from build123d import *

# Parameters (mm, degrees)
SKETCH_1_R             = 7
EXTRUDE_1_DEPTH        = 160
EXTRUDE_1_DEPTH_BACK   = 36
SKETCH_2_R             = 7
EXTRUDE_2_DEPTH        = 8
SKETCH_3_W             = 18
SKETCH_3_H             = 11
EXTRUDE_3_DEPTH        = 15
EXTRUDE_4_DEPTH        = 30
SKETCH_5_W             = 60
SKETCH_5_H             = 40
EXTRUDE_5_DEPTH        = 6
SKETCH_6_W             = 60
SKETCH_6_H             = 6
EXTRUDE_6_DEPTH        = 60
SKETCH_7_W             = 29.455878384
SKETCH_7_H             = 4
EXTRUDE_7_DEPTH        = 8
PATTERN_LINEAR_1_COUNT = 2
PATTERN_LINEAR_1_PITCH = 52


with BuildPart() as part:
    # 草图1 → 凸台-拉伸1 (new body, two sides)
    with BuildSketch(Plane.XY) as extrude_1_sk:
        Circle(SKETCH_1_R)
    extrude(amount=EXTRUDE_1_DEPTH)
    extrude(extrude_1_sk.sketch, amount=-EXTRUDE_1_DEPTH_BACK)

    # 草图2 → 凸台-拉伸2 (add)
    with BuildSketch(Plane(origin=(0, 0, -36), x_dir=(-1, 0, 0), z_dir=(0, 0, -1))):
        Polygon((20, 7.5), (15, 12.5), (-15, 12.5), (-20, 7.5), (-20, -7.5), (-15, -12.5), (15, -12.5), (20, -7.5), align=None)
        Circle(SKETCH_2_R, mode=Mode.SUBTRACT)
        Circle(SKETCH_2_R)
    extrude(amount=EXTRUDE_2_DEPTH)

    # 草图3 → 凸台-拉伸3 (add)
    with BuildSketch(Plane(origin=(0, 0, -44), x_dir=(-1, 0, 0), z_dir=(0, 0, -1))):
        Rectangle(SKETCH_3_W, SKETCH_3_H)
    extrude(amount=EXTRUDE_3_DEPTH)

    # 草图4 → 凸台-拉伸4 (add)
    with BuildSketch(Plane(origin=(0, 0, -59), x_dir=(-1, 0, 0), z_dir=(0, 0, -1))):
        with BuildLine():
            Line((-15, -12.5), (-15, 12.5))
            ThreePointArc((-15, 12.5), (-27.5, 0), (-15, -12.5))
        make_face()
        with BuildLine():
            ThreePointArc((-3.77502784, 5.5), (-8.385621722, 10.606601718), (-15, 12.5))
            Line((-15, 12.5), (-15, -12.5))
            ThreePointArc((-15, -12.5), (-8.385621722, -10.606601718), (-3.77502784, -5.5))
            Line((-3.77502784, -5.5), (-9, -5.5))
            Line((-9, -5.5), (-9, 5.5))
            Line((-9, 5.5), (-3.77502784, 5.5))
        make_face()
        with BuildLine():
            ThreePointArc((-2.5, 0), (-2.822928267, 2.822928267), (-3.77502784, 5.5))
            Line((-3.77502784, 5.5), (-9, 5.5))
            Line((-9, 5.5), (-9, -5.5))
            Line((-9, -5.5), (-3.77502784, -5.5))
            ThreePointArc((-3.77502784, -5.5), (-2.822928267, -2.822928267), (-2.5, 0))
        make_face()
        with BuildLine():
            ThreePointArc((3.77502784, -5.5), (2.5, 0), (3.77502784, 5.5))
            Line((3.77502784, 5.5), (-3.77502784, 5.5))
            ThreePointArc((-3.77502784, 5.5), (-2.822928267, 2.822928267), (-2.5, 0))
            ThreePointArc((-2.5, 0), (-2.822928267, -2.822928267), (-3.77502784, -5.5))
            Line((-3.77502784, -5.5), (3.77502784, -5.5))
        make_face()
        with BuildLine():
            Line((9, 5.5), (3.77502784, 5.5))
            ThreePointArc((3.77502784, 5.5), (2.5, 0), (3.77502784, -5.5))
            Line((3.77502784, -5.5), (9, -5.5))
            Line((9, -5.5), (9, 5.5))
        make_face()
        with BuildLine():
            Line((15, -12.5), (15, 12.5))
            ThreePointArc((15, 12.5), (8.385621722, 10.606601718), (3.77502784, 5.5))
            Line((3.77502784, 5.5), (9, 5.5))
            Line((9, 5.5), (9, -5.5))
            Line((9, -5.5), (3.77502784, -5.5))
            ThreePointArc((3.77502784, -5.5), (8.385621722, -10.606601718), (15, -12.5))
        make_face()
        with BuildLine():
            ThreePointArc((27.5, 0), (23.838834765, 8.838834765), (15, 12.5))
            Line((15, 12.5), (15, -12.5))
            ThreePointArc((15, -12.5), (23.838834765, -8.838834765), (27.5, 0))
        make_face()
        with BuildLine():
            Line((-15, -12.5), (15, -12.5))
            ThreePointArc((15, -12.5), (8.385621722, -10.606601718), (3.77502784, -5.5))
            Line((3.77502784, -5.5), (-3.77502784, -5.5))
            ThreePointArc((-3.77502784, -5.5), (-8.385621722, -10.606601718), (-15, -12.5))
        make_face()
        with BuildLine():
            ThreePointArc((3.77502784, 5.5), (8.385621722, 10.606601718), (15, 12.5))
            Line((15, 12.5), (-15, 12.5))
            ThreePointArc((-15, 12.5), (-8.385621722, 10.606601718), (-3.77502784, 5.5))
            Line((-3.77502784, 5.5), (3.77502784, 5.5))
        make_face()
    extrude(amount=EXTRUDE_4_DEPTH)

    # 草图5 → 凸台-拉伸5 (add)
    with BuildSketch(Plane(origin=(0, 0, -89), x_dir=(-1, 0, 0), z_dir=(0, 0, -1))):
        Rectangle(SKETCH_5_W, SKETCH_5_H)
    extrude(amount=EXTRUDE_5_DEPTH)

    # 草图6 → 凸台-拉伸6 (add)
    with BuildSketch(Plane(origin=(0, 0, -95), x_dir=(-1, 0, 0), z_dir=(0, 0, -1))):
        with Locations((0, 17)):
            Rectangle(SKETCH_6_W, SKETCH_6_H)
        with Locations((0, -17)):
            Rectangle(SKETCH_6_W, SKETCH_6_H)
    extrude(amount=EXTRUDE_6_DEPTH)

    # 草图7 → 凸台-拉伸7 (add)
    with BuildSketch(Plane.ZY.offset(30)):
        Polygon((-125, 8), (-125, 14), (-155, 14), (-160, 14), (-160, 8), align=None)
        Polygon((-125, -8), (-160, -8), (-160, -14), (-155, -14), (-125, -14), align=None)
        Polygon((-160, 8), (-160, 14), (-166, 14), (-166, 4), (-166, 0), (-166, -4), (-166, -14), (-160, -14), (-160, -8), align=None)
        with Locations((-180.727939192, -2)):
            Rectangle(SKETCH_7_W, SKETCH_7_H)
        with Locations((-180.727939192, 2)):
            Rectangle(SKETCH_7_W, SKETCH_7_H)
    extrude_7 = extrude(amount=-EXTRUDE_7_DEPTH)

    # 阵列(线性)1: 凸台-拉伸7 ×2
    with Locations(*[(i * PATTERN_LINEAR_1_PITCH, 0, 0) for i in range(1, PATTERN_LINEAR_1_COUNT)]):
        add(extrude_7)


solid = part.part
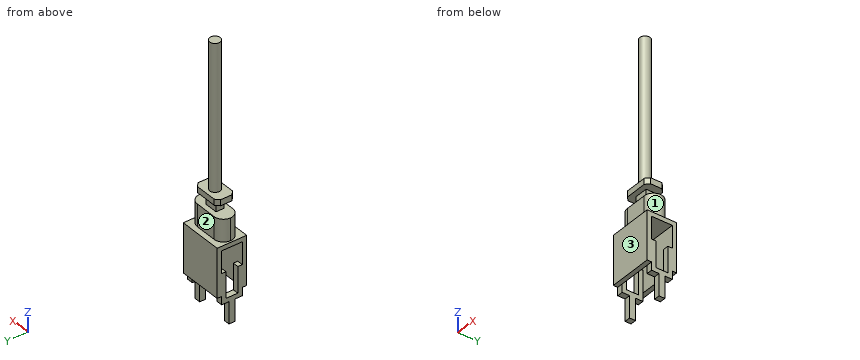
Can you work these out from the model? Positions are in its coordinate system, mm. Face numbers are marked on the shaded views. A direction names the side the tool comes from. Give positions to 0.01 mm unless a question says otherwise; leave off trailing zeros. Loops run counter-clockwise (first coordinate to the right, second up) from the corner with the lowest first, then second, coordinate; pieces in that order, holes last. Notation, with made-up numbers: (76, 62.25) - (130, 62.25) arc R21 ccw to (130, 90.25) - close; hole circle Ø4 at (40, 70). An arc over 180 degrees is marked (long way). Answer as a JSON object with one key per item and string values.
Q1. Which directions (+Z, -Z, +X, -X, +Y, -Y) give clear straight access to the entire face, cutting with the end or side of a thin tool? Please do the marked faces 1, 2 and 3.
Geometry says:
{"face 1": "+Z, +X", "face 2": "+Z, +X, -X, +Y", "face 3": "+Z, -Z, +X, -X, -Y"}
Q2. If I drill on L1, parallel to Y at x = 15, z = -121.5; L2, parallel to Z at x = 14, y = 9; L3, parallel to Z at x = 24.5, y = 1, over which ranges is the centre line in solid material (lowest first)?
Geometry says:
{"L1": "-20 to -14, 14 to 20", "L2": "-95 to -59, -44 to -36", "L3": "-195.46 to -160, -95 to -59"}
Q3. Imagine slicing it at B-B on x = 0. Write out the boundary of the cut face in (y, z), plus the area to 3 significant figures.
Geometry says:
{"outline": "(-20, -155) - (-14, -155) - (-14, -95) - (14, -95) - (14, -155) - (20, -155) - (20, -89) - (12.5, -89) - (12.5, -59) - (5.5, -59) - (5.5, -44) - (12.5, -44) - (12.5, -36) - (7, -36) - (7, 160) - (-7, 160) - (-7, -36) - (-12.5, -36) - (-12.5, -44) - (-5.5, -44) - (-5.5, -59) - (-12.5, -59) - (-12.5, -89) - (-20, -89) - close", "area": "4,820 mm²"}
Q4. Imagine slicing it at C-C on z = 129. Write out the boundary of the cut face in (x, y).
Geometry says:
{"outline": "circle Ø14 at (0, 0)"}
Q5. Will these pins go through, and if not, where does the flat tip stop? P1, Ø2.5, axis at y = 3, z = -41, coming from the -X side; P2, Ø4, axis at x = -26.5, y = 10, coming from the -Z side; P3, Ø12, axis at y = -10, z = 103.5, coming from the +X side.
Geometry says:
{"P1": "x = -20", "P2": "z = -166", "P3": "x = 5.74"}
Q6. Imagine slicing it at A-A on z = -77. Write out the boundary of the cut face in (x, y).
Geometry says:
{"outline": "(-15, -12.5) - (15, -12.5) arc R12.5 ccw to (15, 12.5) - (-15, 12.5) arc R12.5 ccw to start"}
